```python
from build123d import *

# Parameters (mm, degrees)
F1_DEPTH    = 10
F2_T2_ANGLE = 240.9746670828
F2_T4_ANGLE = 240.9746670828
F2_T6_ANGLE = 240.9746670828
F2_T8_ANGLE = 240.9746670828


# Not quite as in the source:
# - a fillet or chamfer that OpenCascade refuses, or shapes differently, is made with other operations: its cross-section is extruded or revolved along the edge and cut away or added


with BuildPart() as f1:
    # F0 (on Top) → F1 (new body)
    with BuildSketch(Plane.XY):
        with BuildLine():
            ThreePointArc((6.3393482774, 11.7357549763), (6.1040734685, 10.1783374237), (6.3649625736, 8.6250053459))
            Line((6.3649625736, 8.6250053459), (8.9305315263, 1))
            Line((8.9305315263, 1), (11.4305315263, 1))
            Line((11.4305315263, 1), (6.7557454084, 14.8937092698))
            ThreePointArc((6.7557454084, 14.8937092698), (6.001778287, 15.1965058009), (5.1958549099, 15.2996545758))
            Line((5.1958549099, 15.2996545758), (0, 15.2996545758))
            Line((0, 15.2996545758), (-5.1958549099, 15.2996545758))
            ThreePointArc((-5.1958549099, 15.2996545758), (-6.001778287, 15.1965058009), (-6.7557454084, 14.8937092698))
            Line((-6.7557454084, 14.8937092698), (-11.4305315263, 1))
            Line((-11.4305315263, 1), (-8.9305315263, 1))
            Line((-8.9305315263, 1), (-6.3649625736, 8.6250053459))
            ThreePointArc((-6.3649625736, 8.6250053459), (-6.1040734685, 10.1783374237), (-6.3393482774, 11.7357549763))
            ThreePointArc((-6.3393482774, 11.7357549763), (-5.3305463755, 13.2920715369), (-4, 12))
            Line((-4, 12), (-5, 0))
            Line((-5, 0), (-5, -17))
            ThreePointArc((-5, -17), (-2.0559445405, -30.8393753001), (6.2663710998, -42.2820512821))
            ThreePointArc((6.2663710998, -42.2820512821), (7.9231903792, -46), (6.2663710998, -49.7179487179))
            ThreePointArc((6.2663710998, -49.7179487179), (-2.0559445405, -61.1606246999), (-5, -75))
            Line((-5, -75), (-5, -92))
            Line((-5, -92), (-4, -104))
            ThreePointArc((-4, -104), (-5.3305463755, -105.2920715369), (-6.3393482774, -103.7357549763))
            ThreePointArc((-6.3393482774, -103.7357549763), (-6.1040734685, -102.1783374237), (-6.3649625736, -100.6250053459))
            Line((-6.3649625736, -100.6250053459), (-8.9305315263, -93))
            Line((-8.9305315263, -93), (-11.4305315263, -93))
            Line((-11.4305315263, -93), (-6.7557454084, -106.8937092698))
            ThreePointArc((-6.7557454084, -106.8937092698), (-6.001778287, -107.1965058009), (-5.1958549099, -107.2996545758))
            Line((-5.1958549099, -107.2996545758), (0, -107.2996545758))
            Line((0, -107.2996545758), (5.1958549099, -107.2996545758))
            ThreePointArc((5.1958549099, -107.2996545758), (6.001778287, -107.1965058009), (6.7557454084, -106.8937092698))
            Line((6.7557454084, -106.8937092698), (11.4305315263, -93))
            Line((11.4305315263, -93), (8.9305315263, -93))
            Line((8.9305315263, -93), (6.3649625736, -100.6250053459))
            ThreePointArc((6.3649625736, -100.6250053459), (6.1040734685, -102.1783374237), (6.3393482774, -103.7357549763))
            ThreePointArc((6.3393482774, -103.7357549763), (5.3305463755, -105.2920715369), (4, -104))
            Line((4, -104), (5, -92))
            Line((5, -92), (5, -75))
            ThreePointArc((5, -75), (29, -51), (53, -75))
            Line((53, -75), (53, -92))
            Line((53, -92), (54, -104))
            ThreePointArc((54, -104), (52.6694536245, -105.2920715369), (51.6606517226, -103.7357549763))
            ThreePointArc((51.6606517226, -103.7357549763), (51.8959265315, -102.1783374237), (51.6350374264, -100.6250053459))
            Line((51.6350374264, -100.6250053459), (49.0694684737, -93))
            Line((49.0694684737, -93), (46.5694684737, -93))
            Line((46.5694684737, -93), (51.2442545916, -106.8937092698))
            ThreePointArc((51.2442545916, -106.8937092698), (51.998221713, -107.1965058009), (52.8041450901, -107.2996545758))
            Line((52.8041450901, -107.2996545758), (58, -107.2996545758))
            Line((58, -107.2996545758), (63.1958549099, -107.2996545758))
            ThreePointArc((63.1958549099, -107.2996545758), (64.001778287, -107.1965058009), (64.7557454084, -106.8937092698))
            Line((64.7557454084, -106.8937092698), (69.4305315263, -93))
            Line((69.4305315263, -93), (66.9305315263, -93))
            Line((66.9305315263, -93), (64.3649625736, -100.6250053459))
            ThreePointArc((64.3649625736, -100.6250053459), (64.1040734685, -102.1783374237), (64.3393482774, -103.7357549763))
            ThreePointArc((64.3393482774, -103.7357549763), (63.3305463755, -105.2920715369), (62, -104))
            Line((62, -104), (63, -92))
            Line((63, -92), (63, -75))
            ThreePointArc((63, -75), (60.0559445405, -61.1606246999), (51.7336289002, -49.7179487179))
            ThreePointArc((51.7336289002, -49.7179487179), (50.0768096208, -46), (51.7336289002, -42.2820512821))
            ThreePointArc((51.7336289002, -42.2820512821), (60.0559445405, -30.8393753001), (63, -17))
            Line((63, -17), (63, 0))
            Line((63, 0), (62, 12))
            ThreePointArc((62, 12), (63.3305463755, 13.2920715369), (64.3393482774, 11.7357549763))
            ThreePointArc((64.3393482774, 11.7357549763), (64.1040734685, 10.1783374237), (64.3649625736, 8.6250053459))
            Line((64.3649625736, 8.6250053459), (66.9305315263, 1))
            Line((66.9305315263, 1), (69.4305315263, 1))
            Line((69.4305315263, 1), (64.7557454084, 14.8937092698))
            ThreePointArc((64.7557454084, 14.8937092698), (64.001778287, 15.1965058009), (63.1958549099, 15.2996545758))
            Line((63.1958549099, 15.2996545758), (58, 15.2996545758))
            Line((58, 15.2996545758), (52.8041450901, 15.2996545758))
            ThreePointArc((52.8041450901, 15.2996545758), (51.998221713, 15.1965058009), (51.2442545916, 14.8937092698))
            Line((51.2442545916, 14.8937092698), (46.5694684737, 1))
            Line((46.5694684737, 1), (49.0694684737, 1))
            Line((49.0694684737, 1), (51.6350374264, 8.6250053459))
            ThreePointArc((51.6350374264, 8.6250053459), (51.8959265315, 10.1783374237), (51.6606517226, 11.7357549763))
            ThreePointArc((51.6606517226, 11.7357549763), (52.6694536245, 13.2920715369), (54, 12))
            Line((54, 12), (53, 0))
            Line((53, 0), (53, -17))
            ThreePointArc((53, -17), (29, -41), (5, -17))
            Line((5, -17), (5, 0))
            Line((5, 0), (4, 12))
            ThreePointArc((4, 12), (5.3305463755, 13.2920715369), (6.3393482774, 11.7357549763))
        make_face()
    extrude(amount=F1_DEPTH)

    # F2: fillet of radius 3 on 4 edges, made by hand

    # F2_s1 → F2_t2 (revolve, cut)
    with BuildSketch(Plane(origin=(14.8970987107, -25.3030447424, 0), x_dir=(0, 0, 1), z_dir=(-0.507347869, 0.8617413416, 0))):
        with BuildLine():
            ThreePointArc((10, 43.3655851338), (9.1213203436, 41.2442647902), (7, 40.3655851338))
            Line((7, 40.3655851338), (10, 40.3655851338))
            Line((10, 40.3655851338), (10, 43.3655851338))
        make_face()
    revolve(axis=Axis((29, -17, 10), (0, 0, -1)), revolution_arc=F2_T2_ANGLE, mode=Mode.SUBTRACT)

    # F2_s3 → F2_t4 (revolve, cut)
    with BuildSketch(Plane(origin=(14.8970987107, -25.3030447424, 0), x_dir=(0, 0, 1), z_dir=(-0.507347869, 0.8617413416, 0))):
        with BuildLine():
            ThreePointArc((3, 40.3655851338), (0.8786796564, 41.2442647902), (0, 43.3655851338))
            Line((0, 43.3655851338), (0, 40.3655851338))
            Line((0, 40.3655851338), (3, 40.3655851338))
        make_face()
    revolve(axis=Axis((29, -17, 0), (0, 0, -1)), revolution_arc=F2_T4_ANGLE, mode=Mode.SUBTRACT)

    # F2_s5 → F2_t6 (revolve, cut)
    with BuildSketch(Plane(origin=(40.2548514411, -68.3737368527, 0), x_dir=(0, 0, 1), z_dir=(0.507347869, -0.8617413416, 0))):
        with BuildLine():
            ThreePointArc((10, 40.0605912676), (9.1213203436, 37.939270924), (7, 37.0605912676))
            Line((7, 37.0605912676), (10, 37.0605912676))
            Line((10, 37.0605912676), (10, 40.0605912676))
        make_face()
    revolve(axis=Axis((29, -75, 10), (0, 0, -1)), revolution_arc=F2_T6_ANGLE, mode=Mode.SUBTRACT)

    # F2_s7 → F2_t8 (revolve, cut)
    with BuildSketch(Plane(origin=(40.2548514411, -68.3737368527, 0), x_dir=(0, 0, 1), z_dir=(0.507347869, -0.8617413416, 0))):
        with BuildLine():
            ThreePointArc((3, 37.0605912676), (0.8786796564, 37.939270924), (0, 40.0605912676))
            Line((0, 40.0605912676), (0, 37.0605912676))
            Line((0, 37.0605912676), (3, 37.0605912676))
        make_face()
    revolve(axis=Axis((29, -75, 0), (0, 0, -1)), revolution_arc=F2_T8_ANGLE, mode=Mode.SUBTRACT)


solid = f1.part
```
Build history of the part. All positions in model axes, mm. A direction names the side the tool comes from. Round coordinates to 2 decimals unless told otherwise and drop trailing zeros. Write each loop counter-clockwise with the first axis right and the second up, starting at its lowest first coordinate (ties: lowest second). Pieces come first, ordered by that corner, then holes.
1) Band-saw the part on B-B, the plane y = -98. List the corners of the cut face in (x, z), and give its area (3 significant figures).
2) Band-saw the part on A-A, the plane x = 29. List the corners of the cut face in (y, z).
3) Mould opens along Y. For faces 1 (the cylindrical face through (60.137, -61.343, 4.93)), 2 (the flat face through (0, 15.3, 5)), 3 (the flat face through (29, -46, 10)) say: +Y half, -Y half, draft (parallel to the pull), parting line (faces both ways), or undercut.
4) Drill centre lines: probe 1 along X at (y, z) = (-7, 5.5); probe 2 along X at (y, z) = (-46, 5); probe 3 along X at (y, z) = (-64.5, 4.25). Where is each one in solid material? Low to high.
5) Pin check, flat tips, straight feed: pin 1 (3 mm diameter, centred on x = 13.5, z = 3, fed in from +Y); pin 2 (3 mm diameter, centred on y = -4.5, z = 3.5, fed in from +X); pin 3 (5 mm diameter, centred on y = -9.5, z = 7, fed in from -X); pin 4 (3 mm diameter, centred on x = 63.2, y = -104.1, fed in from +Z). Stop position of each tip, or through.
6) 3-axis set-ups, long thin cutter, end or side, ignore diameter. For faces 4 (the flat face through (63, -84, 5)), 5 (the cylindrical face through (-6.104, 10.156, 4.93)), 6 (the flat face through (-5, -83, 5)), 7 (the flat face through (-9.06, 8.04, 4.93)): which of +Z, -Z, +X, -X, +Y, -Y reach the whole face in a straight line?
Ans:
1. outline: (-9.75, 0) - (-7.25, 0) - (-7.25, 10) - (-9.75, 10) - close; (-4.5, 0) - (4.5, 0) - (4.5, 10) - (-4.5, 10) - close; (7.25, 0) - (9.75, 0) - (9.75, 10) - (7.25, 10) - close; (48.25, 0) - (50.75, 0) - (50.75, 10) - (48.25, 10) - close; (53.5, 0) - (62.5, 0) - (62.5, 10) - (53.5, 10) - close; (65.25, 0) - (67.75, 0) - (67.75, 10) - (65.25, 10) - close
1. area: 280 mm2
2. outline: (-51, 3) arc R3 ccw to (-48, 0) - (-44, 0) arc R3 ccw to (-41, 3) - (-41, 7) arc R3 ccw to (-44, 10) - (-48, 10) arc R3 ccw to (-51, 7) - close
3. face 1: undercut
3. face 2: +Y half
3. face 3: draft
4. probe 1: x = -5 to 5, 53 to 63
4. probe 2: x = 7.92 to 50.08
4. probe 3: x = -3.34 to 7.42, 50.58 to 61.34
5. pin 1: stops at y = -33.94
5. pin 2: stops at x = 63
5. pin 3: stops at x = -5
5. pin 4: stops at z = 10
6. face 4: +Z, -Z, +X
6. face 5: +Z, -Z
6. face 6: +Z, -Z, -X
6. face 7: +Z, -Z, -X, +Y
